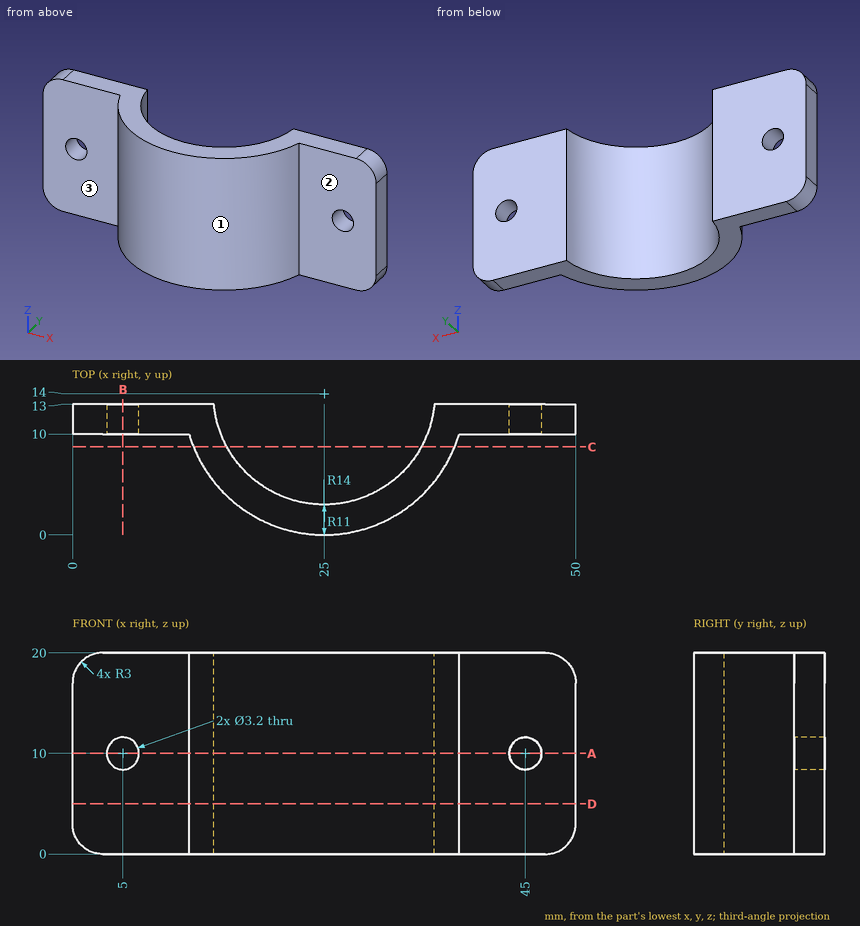
Can you work these out from the drawing? Everything is in mm from the part's minimum corner. A direction names the side the tool comes from. Coordinates: 2 decimals unless noted, no trailing zeros. Write each loop counter-clockwise with the first axis right and the second up, starting at its lowest first coordinate (ties: lowest second). Pieces come first, ordered by that corner, then holes. Notation, with made-up numbers: (54.25, 31.25) - (112.25, 31.25) arc R18 ccw to (112.25, 44.25) - close; hole circle Ø2 at (-16, 15.25). An arc over 180 degrees is marked (long way). Use a Markdown table: item, result.
Q1. I'm going to push flat-ended pins straight in: pin 1 Ø4 at (y, z) = (1.5, 16) entering from +X; pin 2 Ø12 at (x, z) = (29, 5) entering from +Y; pin 3 Ø3.5 at (x, z) = (43, 6.5) entering from -Y. Where does each tip first touch, or does it pass through?
Geometry check:
| item | result |
|---|---|
| pin 1 | stops at x = 34.26 |
| pin 2 | stops at y = 9.42 |
| pin 3 | stops at y = 10 |
Q2. Which directions (+Z, -Z, +X, -X, +Y, -Y) give clear straight access to the entire face, cutting with the end or side of a thin tool? Please do the marked faces 1, 2 and 3.
Geometry check:
| item | result |
|---|---|
| face 1 | +Z, -Z, -Y |
| face 2 | +Z, -Z, +X, -Y |
| face 3 | +Z, -Z, -X, -Y |
Q3. Imagine slicing it at D-D (z = 5). List the corners of the cut face in (x, y) for me.
Geometry check:
| item | result |
|---|---|
| outline | (0, 10) - (11.58, 10) arc R14 ccw to (38.42, 10) - (50, 10) - (50, 13) - (35.95, 13) arc R11 cw to (14.05, 13) - (0, 13) - close |
Q4. Please list where these lines run through material, in increasing order: L1, parallel to Z at x = 5, y = 11.8; L2, parallel to X at y = 10.5, z = 11.25; L3, parallel to Y at x = 39.5, z = 1.5.
Geometry check:
| item | result |
|---|---|
| L1 | z = 0 to 8.4, 11.6 to 20 |
| L2 | x = 0 to 4, 6 to 14.57, 35.43 to 44, 46 to 50 |
| L3 | y = 10 to 13 |
Q5. Imagine slicing it at C-C (y = 8.75). List the corners of the cut face in (x, z) for me, and give its area (3 significant figures).
Geometry check:
| item | result |
|---|---|
| outline | (12.02, 0) - (15.33, 0) - (15.33, 20) - (12.02, 20) - close; (34.67, 0) - (37.98, 0) - (37.98, 20) - (34.67, 20) - close |
| area | 132 mm2 |
Q6. Imagine slicing it at B-B (x = 5). List the corners of the cut face in (y, z) for me, and give its area (3 significant figures).
Geometry check:
| item | result |
|---|---|
| outline | (10, 0) - (13, 0) - (13, 8.4) - (10, 8.4) - close; (10, 11.6) - (13, 11.6) - (13, 20) - (10, 20) - close |
| area | 50.4 mm2 |
Q7. Imagine slicing it at A-A (z = 10). List the corners of the cut face in (x, y) for me.
Geometry check:
| item | result |
|---|---|
| outline | (0, 10) - (3.4, 10) - (3.4, 13) - (0, 13) - close; (6.6, 10) - (11.58, 10) arc R14 ccw to (38.42, 10) - (43.4, 10) - (43.4, 13) - (35.95, 13) arc R11 cw to (14.05, 13) - (6.6, 13) - close; (46.6, 10) - (50, 10) - (50, 13) - (46.6, 13) - close |
